Answer from the drawing. Dimensions are ordinates in mm from the lowest x, y and z of the part. A direction names the side the tool comes from. Give positions to 0.01 mm unless a question says otherwise; leave off trailing zeros. Loops run counter-clockwise (first coordinate to the right, second up) from the corner with the lowest first, then second, coordinate; pieces in that order, holes last.
(1) Each of these flat-tipped pins is pushed along its axis until it touches: P1, Ø14.5, axis at x = 95, y = 20, coming from the +Z side; P2, Ø8, axis at y = 35.5, z = 33, coming from the -X side; P3, Ø12, axis at y = 36, z = 48.5, coming from the +X side; P4, Ø6.5, axis at x = 95, y = 20, coming from the +Z side. Where does it stop, or does it pass through?
(2) Find section D-D, the plane z = 43. Write down the section's boundary in (x, y), then the cut area to 3 significant figures.
(3) Find section A-A, the plane y = 20. Write down the section's boundary in (x, z).
(4) Determine the mould class of the marked faces 1, 2 and 3 for opening direction Y: pulls with the +Y half, pulls with the -Y half, needs draft (parallel to the pull), parting line crosses it, or undercut.
(5) Straight lines are drawn through the part: probe 1 along Y at (x, z) = (15, 12); probe 2 along Y at (x, z) = (95, 4); probe 3 along X at (y, z) = (12, 9.5). For each, find the intervals that lie inside material, in ascending order.
(6) Which of the six approach directions +Z, -Z, +X, -X, +Y, -Y give full straight-line access (tool end or side, diameter ignored) to the marked faces 4, 5, 6 and 7?
(7) Find section B-B, the plane x = 15. Write down the section's boundary in (y, z).
(8) Find section C-C, the plane z = 11.5. Write down the section's boundary in (x, y), then the cut area to 3 significant figures.
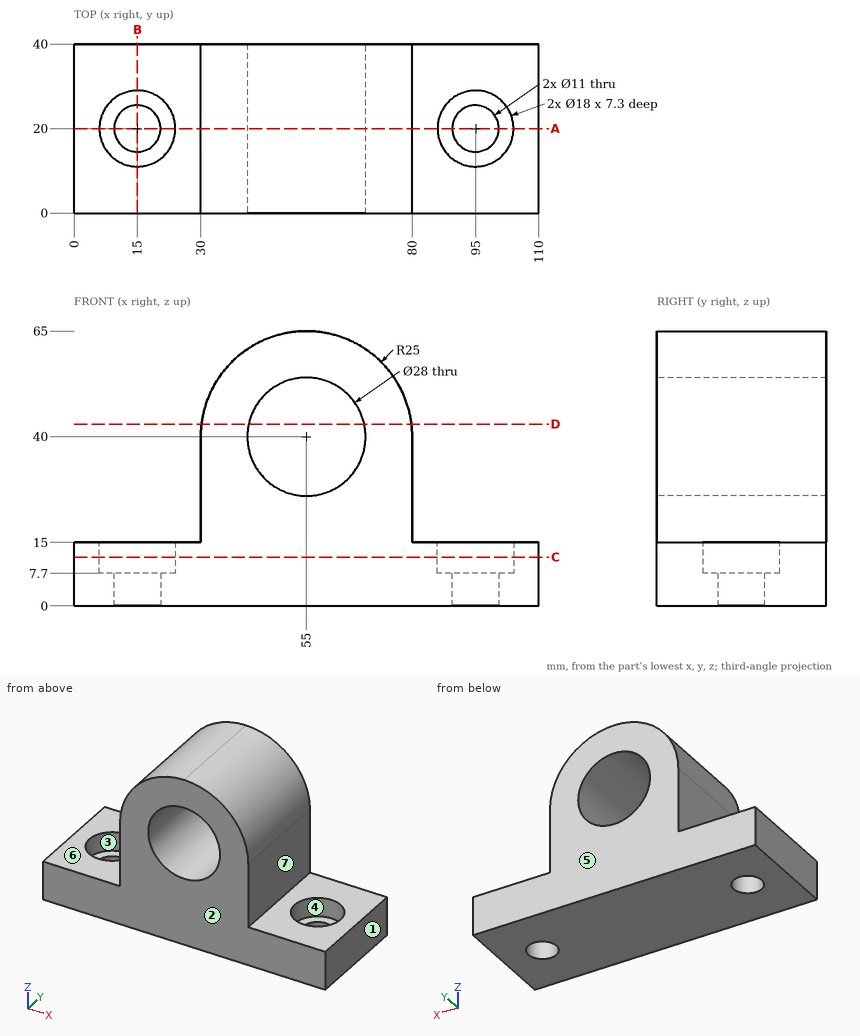
Entries:
1. P1: stops at z = 7.7
1. P2: stops at x = 30
1. P3: stops at x = 79.87
1. P4: passes through
2. outline: (30.18, 0) - (41.33, 0) - (41.33, 40) - (30.18, 40) - close; (68.67, 0) - (79.82, 0) - (79.82, 40) - (68.67, 40) - close
2. area: 892 mm2
3. outline: (0, 0) - (9.5, 0) - (9.5, 7.7) - (6, 7.7) - (6, 15) - (0, 15) - close; (20.5, 0) - (89.5, 0) - (89.5, 7.7) - (86, 7.7) - (86, 15) - (80, 15) - (80, 40) arc R25 ccw to (55, 65) arc R25 ccw to (30, 40) - (30, 15) - (24, 15) - (24, 7.7) - (20.5, 7.7) - close; (100.5, 0) - (110, 0) - (110, 15) - (104, 15) - (104, 7.7) - (100.5, 7.7) - close; hole circle Ø28 at (55, 40)
4. face 1: needs draft
4. face 2: pulls with the -Y half
4. face 3: undercut
5. probe 1: y = 0 to 11, 29 to 40
5. probe 2: y = 0 to 14.5, 25.5 to 40
5. probe 3: x = 0 to 10.88, 19.12 to 90.88, 99.12 to 110
6. face 4: +Z
6. face 5: +Z, -Z, +X, -X, +Y
6. face 6: +Z, -X, +Y, -Y
6. face 7: +Z, +X, +Y, -Y
7. outline: (0, 0) - (14.5, 0) - (14.5, 7.7) - (11, 7.7) - (11, 15) - (0, 15) - close; (25.5, 0) - (40, 0) - (40, 15) - (29, 15) - (29, 7.7) - (25.5, 7.7) - close
8. outline: (0, 0) - (110, 0) - (110, 40) - (0, 40) - close; hole circle Ø18 at (15, 20); hole circle Ø18 at (95, 20)
8. area: 3,890 mm2
